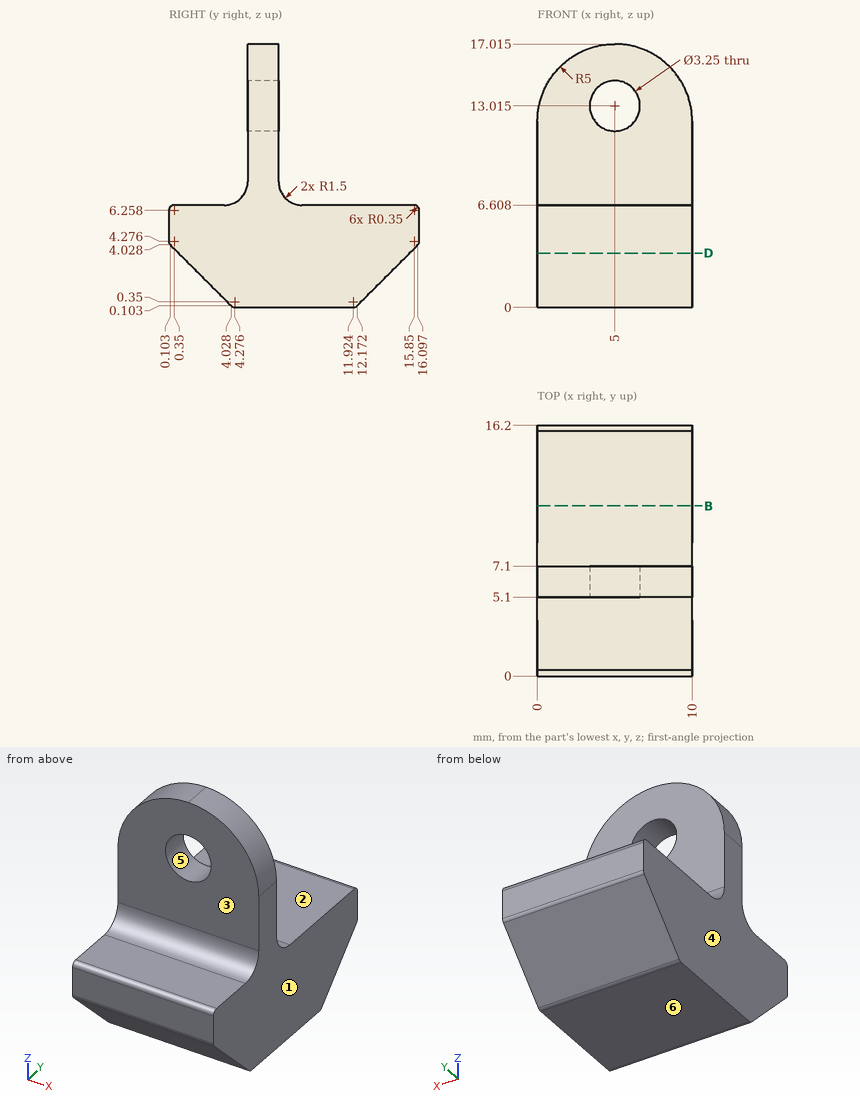
Verification items for this drawing (mm, ordinates from the low corner). A direction names the side the tool comes from. Round coordinates to 2 decimals unless told otherwise and drop trailing zeros. Order: outer loops, then holes, each group sorted by start corner. A loop starts at its lowest first (then second) coordinate and runs counter-clockwise, first axis right, second up. Notation, with made-up numbers: M 27,52.25 L 39,52.25 A28 cw 39,85.25 Z; hole C 46,51 d3. An arc over 180 degrees is marked long. Answer in a Markdown table with one row per item. Add a question column.
Item 1: Sectioned sample at D-D, the plane z = 3.5. Enter the section's corners in (x, y).
Item 2: Draft check along X on the marked faces 4, 5 and 6. Enter one of: released by +X, released by -X, zero draft, split by the parting line, or undercut.
Item 3: Set-up check for the marked faces 1, 2 and 3: record each of +Z, -Z, +X, -X, +Y, -Y from which the full face is reachable in a straight line by a thin tool's end or side.
Item 4: Sectioned sample at B-B, the plane y = 11. Enter the section's corners in (x, z).
Item 5: Depth check by flat-ended pin: pin 1 Ø5 at (x, z) = (6, 12) entering from -Y; pin 2 Ø6 at (y, z) = (13.5, 11) entering from -X; pin 3 Ø2 at (x, y) = (4.5, 13) entering from +Z; pin 4 Ø4 at (x, z) = (5, 11) entering from +Y. Enter the tip coordinate at first touch or a pass-through.
Item 6: Material ranges on L1, parallel to Z at x = 5, y = 6.15 (1 decimal); L2, parallel to Y at x = 9.5, z = 9.25; L3, parallel to Z at x = 3.75, y = 7.5 (1 decimal), recorded low to high. Write a range as [from, to].
Filled in:
| question | item | result |
|---|---|---|
| 1 | outline | M 0,0.63 L 10,0.63 L 10,15.57 L 0,15.57 Z |
| 2 | face 4 | released by -X |
| 2 | face 5 | undercut |
| 2 | face 6 | zero draft |
| 3 | face 1 | +Z, -Z, +X, +Y, -Y |
| 3 | face 2 | +Z, +X, -X, +Y |
| 3 | face 3 | +Z, +X, -X, -Y |
| 4 | outline | M 0,0 L 10,0 L 10,6.61 L 0,6.61 Z |
| 5 | pin 1 | stops at y = 5.1 |
| 5 | pin 2 | passes through |
| 5 | pin 3 | stops at z = 6.61 |
| 5 | pin 4 | stops at y = 7.1 |
| 6 | L1 | z = [0, 11.4], [14.6, 17] |
| 6 | L2 | y = [5.1, 7.1] |
| 6 | L3 | z = [0, 7.1] |
